Autodesk Inventor part; units mm, degrees
ref_plane "YZ Plane" through (0, 0, 0) normal (1, 0, 0) x (0, 1, 0)
ref_plane "XZ Plane" through (0, 0, 0) normal (0, 1, 0) x (-1, 0, 0)
ref_plane "XY Plane" through (0, 0, 0) normal (0, 0, 1) x (1, 0, 0)
sketch "Sketch1" plane through (0, 0, 0) normal (0, 1, 0) x (-1, 0, 0)
  line L0 (60.86, 0) -> (0, 0)
  line L1 (0, 0) -> (0, -78.39)
  line L2 (0, -78.39) -> (60.86, -78.39)
  line L3 (60.86, -78.39) -> (60.86, 0)
  dimension "d0" = 78.39
  dimension "d1" = 60.86
extrude "Extrusion1" add sketch "Sketch1" along normal blind 2
sketch "Sketch2" plane through (0, 2, 0) normal (0, 1, 0) x (1, 0, 0)
  line L0 (0, 78.39) -> (-60.86, 78.39)
  line L1 (-60.86, 78.39) -> (-60.86, 0)
  point P0 (0, 0)
  point P1 (-30.43, 39.195)
  dimension "d4" = 39.195
  dimension "d5" = 30.43
hole "Hole1" at (-30.43, 2, -39.195) direction (0, -1, 0) diameter 10 end through all
properties part number "pcbProtectiveCaseTop"
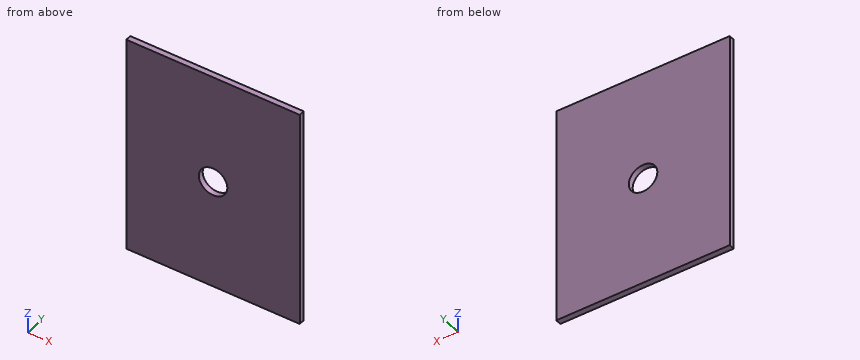
The listing builds one solid part. Answer for the finished solid, in the listing's coordinates (mm). Round coordinates to 2 decimals unless told otherwise and drop trailing zeros. Loops run counter-clockwise (first coordinate to the right, second up) from the corner with the lowest first, then second, coordinate; pieces in that order, holes last. Notation, with made-up numbers: (3.25, 79) - (22.25, 79) arc R25 ccw to (22.25, 115) - close; hole circle Ø4 at (50.5, 36.5). An arc over 180 degrees is marked (long way). Use one line per item in the form item = value. Start each with the question number.
1. Consider line 1 (Z direction, x = -30.43, y = 1) (3 decimals); line 2 (X direction, y = 0.8, z = -39); line 3 (Z direction, x = -34.5, y = 1.9). Determine where each line is inside the solid, lowest interval first. Write a range as [from, to].
2. The part is cut by section B-B on y = 1.3. Determine the outline of the cut face in (x, z) (3 decimals), then the cut area to 3 significant figures.
3. Given pin 1 Ø9 at (x, z) = (-30.43, -39.195) entering from +Y, flat-ended and moving along its own axis, determine where the tip first touches the part or whether it passes through.
4. The part is cut by section A-A on x = -30.43. Determine the outline of the cut face in (y, z) (3 decimals).
Geometry check:
q1.line_1 = [-78.39, -44.195], [-34.195, 0]
q1.line_2 = [-60.86, -35.43], [-25.43, 0]
q1.line_3 = [-78.39, -42.1], [-36.29, 0]
q2.outline = (-60.86, -78.39) - (0, -78.39) - (0, 0) - (-60.86, 0) - close; hole circle Ø10 at (-30.43, -39.195)
q2.area = 4,690 mm^2
q3.pin_1 = through
q4.outline = (0, -78.39) - (2, -78.39) - (2, -44.195) - (0, -44.195) - close; (0, -34.195) - (2, -34.195) - (2, 0) - (0, 0) - close
